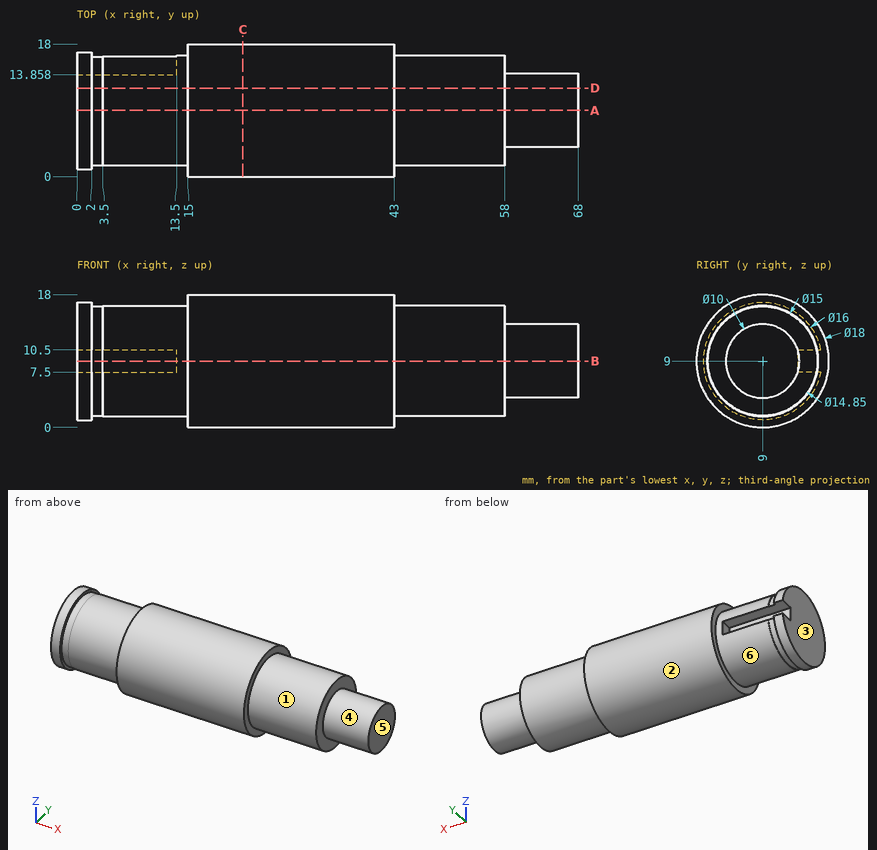
Verification items for this drawing (mm, ordinates from the low corner). A direction names the side the tool comes from. Coordinates: 2 decimals unless noted, no trailing zeros. Loops run counter-clockwise (first coordinate to the right, second up) from the corner with the lowest first, then second, coordinate; pieces in that order, holes last.
Item 1: Sectioned sample at D-D, the plane y = 12. Record the boundary of the cut face in (x, z).
Item 2: Sectioned sample at A-A, the plane y = 9. Record the boundary of the cut face in (x, z) (3 decimals).
Item 3: Release check for a two-part mould opening along X. For the marked faces 3, 4, 5 and 6 record: released by +X, released by -X, zero draft, split by the parting line, or undercut.
Item 4: Sectioned sample at B-B, the plane z = 9. Record the boundary of the cut face in (x, y) (3 decimals), then the cut area to 3 significant figures.
Item 5: Sectioned sample at C-C, the plane x = 22.5. Record the boundary of the cut face in (y, z), then the cut area to 3 significant figures.
Item 6: Access from +Z, -Z, +X, -X, +Y, -Y to the whole of each face (thin tool, end or side, straight path). Record for the marked faces 1 and 2.
Item 7: Thickness scan on line 1 (X direction, y = 8, z = 4); line 2 (Z direction, x = 14.5, y = 9); line 3 (Z direction, x = 25, y = 9.25). Record the ranges inside material, lowest first.
Item 8: Go/stop test with flat-tipped pins: pin 1 Ø2.5 at (x, z) = (6, 9.5) entering from +Y; pin 2 Ø3.5 at (x, y) = (4.5, 15) entering from +Z; pin 3 Ø5 at (x, y) = (33, 13.5) entering from +Z (3 decimals). Record where each tip stops, or that it passes through.
Check result:
1. outline: (0, 1.58) - (2, 1.58) - (2, 2.21) - (3.5, 2.21) - (3.5, 2.13) - (15, 2.13) - (15, 0.51) - (43, 0.51) - (43, 2.13) - (58, 2.13) - (58, 5) - (68, 5) - (68, 13) - (58, 13) - (58, 15.87) - (43, 15.87) - (43, 17.49) - (15, 17.49) - (15, 15.87) - (3.5, 15.87) - (3.5, 15.79) - (2, 15.79) - (2, 16.42) - (0, 16.42) - close
2. outline: (0, 1) - (2, 1) - (2, 1.575) - (3.5, 1.575) - (3.5, 1.5) - (15, 1.5) - (15, 0) - (43, 0) - (43, 1.5) - (58, 1.5) - (58, 4) - (68, 4) - (68, 14) - (58, 14) - (58, 16.5) - (43, 16.5) - (43, 18) - (15, 18) - (15, 16.5) - (3.5, 16.5) - (3.5, 16.425) - (2, 16.425) - (2, 17) - (0, 17) - close
3. face 3: released by -X
3. face 4: zero draft
3. face 5: released by +X
3. face 6: undercut
4. outline: (0, 1) - (2, 1) - (2, 1.575) - (3.5, 1.575) - (3.5, 1.5) - (15, 1.5) - (15, 0) - (43, 0) - (43, 1.5) - (58, 1.5) - (58, 4) - (68, 4) - (68, 14) - (58, 14) - (58, 16.5) - (43, 16.5) - (43, 18) - (15, 18) - (15, 16.5) - (13.5, 16.5) - (13.5, 13.858) - (0, 13.858) - close
4. area: 1,020 mm2
5. outline: circle Ø18 at (9, 9)
5. area: 254 mm2
6. face 1: +X
6. face 2: +X, -X
7. line 1: x = 0 to 58
7. line 2: z = 1.5 to 16.5
7. line 3: z = 0 to 18
8. pin 1: stops at y = 16.35
8. pin 2: stops at z = 15.18
8. pin 3: stops at z = 17.775
